Source: CAD feature listing. Evaluate the final solid. Frame: model axes, mm. A direction names the side the tool comes from. Coordinates: 2 decimals unless noted, no trailing zeros. Loops run counter-clockwise (first coordinate to the right, second up) from the corner with the lowest first, then second, coordinate; pieces in that order, holes last.
Autodesk Inventor part; units mm, degrees
ref_plane "YZ Plane" through (0, 0, 0) normal (1, 0, 0) x (0, 1, 0)
ref_plane "XZ Plane" through (0, 0, 0) normal (0, 1, 0) x (-1, 0, 0)
ref_plane "XY Plane" through (0, 0, 0) normal (0, 0, 1) x (1, 0, 0)
sketch "Skizze1" plane through (0, 0, 0) normal (0, 0, 1) x (1, 0, 0)
  circle A0 centre (0, 0) radius 25.05 construction
  arc A1 (28.7396, -43.3579) -> (0, 27.05) centre (0, -14.0195) ccw
  circle A2 centre (0, 0) radius 23.1 construction
  line L0 (0, 25.05) -> (0, 23.1)
  arc A3 (25.9755, -40.5362) -> (0, 23.1) centre (0, -14.0195) ccw
  line L1 (0, -63.4548) -> (0, 53.3986) construction
  line L2 (0, -25.05) -> (0, -23.1)
  line L3 (2.0133, -23.0121) -> (2.3576, -26.9471)
  arc A4 (0, 27.05) -> (2.3576, -26.9471) centre (0, 0) ccw
  arc A5 (0, -23.1) -> (2.0133, -23.0121) centre (0, 0) ccw
  arc A6 (0, 25.05) -> (0, -25.05) centre (0, 0) ccw
  arc A7 (25.9755, -40.5362) -> (28.7396, -43.3579) centre (27.3576, -41.9471) ccw
  arc A8 (3.0076, -22.9034) -> (0, 23.1) centre (0, 0) ccw
  line L4 (3.0076, -22.9034) -> (3.3521, -26.8415)
  circle A9 centre (0, 0) radius 27.05 construction
  arc A10 (25.4302, -42.3783) -> (3.3521, -26.8415) centre (5.8399, -46.7614) ccw
  dimension "d0" = 50.1
  dimension "d2" = 46.2
  dimension "d3" = 2
  dimension "d4" = 5
  dimension "d11" = 25
  dimension "d12" = 15
  dimension "d16" = 1
extrude "Extrusion1" add sketch "Skizze1" along normal blind 75 contours A7 A3 L0 A6 L2 A5 L3 A4 A1
equation "\"d0\" = ht_diameter + gap_fit"
equation "\"d2\" = ht_diameter - 2 * ht_thickness"
equation "\"kg_thickness\" = 4.9"
equation "\"ht_diameter\" = 50"
equation "\"ht_thickness\" = 1.9"
equation "\"case_thickness\" = 18"
equation "\"gap_fit\" = 0.1"
equation "\"gap_slide\" = 0.2"
equation "\"gap_air\" = 1"
equation "\"bore_diameter\" = 73"
equation "\"tape_thickness\" = 3"
equation "\"tape_width\" = 15"
equation "\"mdf_thickness\" = 6"
equation "\"inner_thickness\" = 15"
equation "\"inner_depth\" = 255"
properties part number "Züklon_Lufteinlass"
Q1. Section B-B, the plane y = -6.5. Return the cut outline in (x, z).
Q2. Contact query for flat-ended pins moving along their axis: pin 1 Ø0.6 at (y, z) = (24, 55) entering from -X; pin 2 Ø10 at (y, z) = (5, 10.5) entering from +X; pin 3 Ø10 at (y, z) = (3.5, 24) entering from -X. Output: stop coordinate, or through.
Q3. Draft query along Y for faces 3 (the cylindrical face through (-26.99, -1.79, 36.98)), 4 (the flat face through (30, 10, 75)), 5 (the flat face through (2.183, -24.952, 36.975)), 6 (the cylindrical face through (34.13, 0.58, 36.98)). Return one class per face: +Y half, -Y half, draft (parallel to the pull), parting line (faces both ways), or undercut.
Q4. Section C-C, the plane z = 7. Return the cut outline in (x, y).
Q5. Access query for faces 1 (the flat face through (0, 24, 37)), 2 (the flat face through (30, 10, 0)). Directions: +Z, -Z, +X, -X, +Y, -Y. A direction counts if a zero-diameter tool reaches every point of the face in a straight line with its end or side. Return the directions, or none.
Q6. Section D-D, the plane y = -31.5. Return the cut outline in (x, z).
Q7. Section A-A, the plane y = 20. Return the cut outline in (x, z), plus the area to 3 significant figures.
Q8. Line query: line 1 along Y through (x, z) = (-13, 52); line 2 along X through (y, z) = (2, 39); line 3 along X through (y, z) = (14, 20). Output: solid intervals per line, ascending.
Derived:
1. outline: (-26.26, 0) - (-24.19, 0) - (-24.19, 75) - (-26.26, 75) - close; (36.35, 0) - (40.38, 0) - (40.38, 75) - (36.35, 75) - close
2. pin 1: stops at x = -13.04
2. pin 2: stops at x = 38.6
2. pin 3: stops at x = -27.05
3. face 3: parting line
3. face 4: draft
3. face 5: undercut
3. face 6: undercut
4. outline: (0, -25.05) arc R25.05 cw to (0, 25.05) - (0, 23.1) arc R37.12 cw to (25.98, -40.54) arc R1.97 ccw to (28.74, -43.36) arc R41.07 ccw to (0, 27.05) arc R27.05 ccw (long way) to (2.36, -26.95) - (2.01, -23.01) arc R23.1 cw to (0, -23.1) - close
5. face 1: +Z, -Z
5. face 2: -Z, +X, -X, +Y, -Y
6. outline: (32.75, 0) - (37.16, 0) - (37.16, 75) - (32.75, 75) - close
7. outline: (-18.21, 0) - (-15.08, 0) - (-15.08, 75) - (-18.21, 75) - close; (14.85, 0) - (23.01, 0) - (23.01, 75) - (14.85, 75) - close
7. area: 847 mm2
8. line 1: y = -23.72 to -21.41, 21.41 to 23.72
8. line 2: x = -26.98 to -24.97, 33.48 to 37.82
8. line 3: x = -23.15 to -20.77, 24.35 to 30.03
